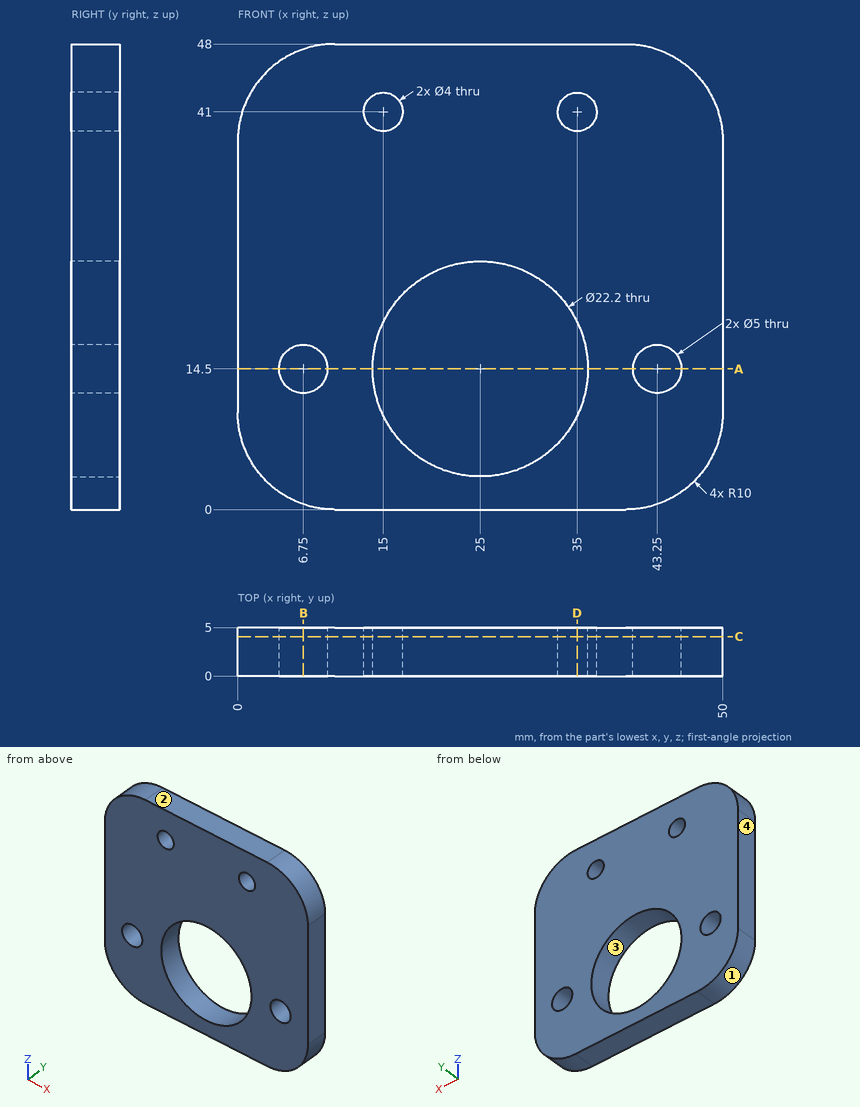
Study the drawing (mm; zero at the part's minimum x, y, z) and answer. Coordinates: 2 decimals unless noted, no trailing zeros. Write each loop counter-clockwise with the first axis right and the second up, starting at its lowest first coordinate (ties: lowest second). Pieces come first, ordered by that corner, then holes. Notation, with made-up numbers: M -31,-18 L 23,-18 A21 cw 23,-6 Z; hole C -22.5,-25.5 d11. An arc over 180 degrees is marked long. Use a Markdown table: item, result. Add a question column.
1. For a pull along Z with two mould halves and no side action, classify the marked faces 1, 2, 3 and 4 as +Z half, -Z half, draft (parallel to the pull), parting line (faces both ways), or undercut.
2. Given P1, Ø1.5, axis at y = 0.5, z = 9.5, coming from the +X side, flat-ended and moving along its own axis, determine where the tip first touches the part or whether it passes through.
3. Section C-C (y = 4.05) is taken. Give the vertices of the cut face in (x, z), plus the area to 3 significant figures.
4. Section D-D (x = 35) is taken. Give the vertices of the cut face in (y, z), plus the area to 3 significant figures.
5. Straight lines are drawn through the part: line 1 along X through (y, z) = (2.65, 14.5); line 2 along X through (y, z) = (1.8, 41); line 3 along X through (y, z) = (4.7, 15.5). For each, find the intervals that lie inside material, in ascending order. Write a range as [from, to].
6. Section A-A (z = 14.5) is taken. Give the vertices of the cut face in (x, y), plus the area to 3 significant figures.
7. Section B-B (x = 6.75) is taken. Give the vertices of the cut face in (y, z).
Data:
| question | item | result |
|---|---|---|
| 1 | face 1 | -Z half |
| 1 | face 2 | +Z half |
| 1 | face 3 | undercut |
| 1 | face 4 | draft |
| 2 | P1 | stops at x = 50 |
| 3 | outline | M 0,10 A10 ccw 10,0 L 40,0 A10 ccw 50,10 L 50,38 A10 ccw 40,48 L 10,48 A10 ccw 0,38 Z; hole C 6.75,14.5 d5; hole C 15,41 d4; hole C 25,14.5 d22.2; hole C 35,41 d4; hole C 43.25,14.5 d5 |
| 3 | area | 1,860 mm2 |
| 4 | outline | M 0,0 L 5,0 L 5,9.68 L 0,9.68 Z; M 0,19.32 L 5,19.32 L 5,39 L 0,39 Z; M 0,43 L 5,43 L 5,48 L 0,48 Z |
| 4 | area | 172 mm2 |
| 5 | line 1 | x = [0, 4.25], [9.25, 13.9], [36.1, 40.75], [45.75, 50] |
| 5 | line 2 | x = [0.46, 13], [17, 33], [37, 49.54] |
| 5 | line 3 | x = [0, 4.46], [9.04, 13.95], [36.05, 40.96], [45.54, 50] |
| 6 | outline | M 0,0 L 4.25,0 L 4.25,5 L 0,5 Z; M 9.25,0 L 13.9,0 L 13.9,5 L 9.25,5 Z; M 36.1,0 L 40.75,0 L 40.75,5 L 36.1,5 Z; M 45.75,0 L 50,0 L 50,5 L 45.75,5 Z |
| 6 | area | 89.0 mm2 |
| 7 | outline | M 0,0.54 L 5,0.54 L 5,12 L 0,12 Z; M 0,17 L 5,17 L 5,47.46 L 0,47.46 Z |
